```python
from build123d import *

# Parameters (mm, degrees)
BOSS_EXTRUDE1_DEPTH = 1828.8
THRU_HOLES_D        = 2.794


with BuildPart() as part:
    # Sketch1 → Boss-Extrude1 (new body)
    with BuildSketch(Plane(origin=(0, 0, 0), x_dir=(1, 0, 0), z_dir=(0, 1, 0))):
        with BuildLine():
            Line((-3.048, 13.208), (-3.048, 4.953))
            ThreePointArc((-3.048, 4.953), (-3.085197439, 4.863197439), (-3.175, 4.826))
            Line((-3.175, 4.826), (-4.826, 4.826))
            ThreePointArc((-4.826, 4.826), (-5.005605122, 4.751605122), (-5.08, 4.572))
            Line((-5.08, 4.572), (-5.08, 0))
            ThreePointArc((-5.08, 0), (-3.592102448, -3.592102448), (0, -5.08))
            Line((0, -5.08), (4.572, -5.08))
            ThreePointArc((4.572, -5.08), (4.751605122, -5.005605122), (4.826, -4.826))
            Line((4.826, -4.826), (4.826, -3.175))
            ThreePointArc((4.826, -3.175), (4.863197439, -3.085197439), (4.953, -3.048))
            Line((4.953, -3.048), (13.208, -3.048))
            ThreePointArc((13.208, -3.048), (13.746815367, -2.824815367), (13.97, -2.286))
            Line((13.97, -2.286), (13.97, 0.508))
            ThreePointArc((13.97, 0.508), (13.746815367, 1.046815367), (13.208, 1.27))
            Line((13.208, 1.27), (3.767428831, 1.27))
            ThreePointArc((3.767428831, 1.27), (3.625438515, 1.313394326), (3.531964529, 1.42875))
            ThreePointArc((3.531964529, 1.42875), (2.694076836, 2.694076836), (1.42875, 3.531964529))
            ThreePointArc((1.42875, 3.531964529), (1.313394326, 3.625438515), (1.27, 3.767428831))
            Line((1.27, 3.767428831), (1.27, 13.208))
            ThreePointArc((1.27, 13.208), (1.046815367, 13.746815367), (0.508, 13.97))
            Line((0.508, 13.97), (-2.286, 13.97))
            ThreePointArc((-2.286, 13.97), (-2.824815367, 13.746815367), (-3.048, 13.208))
        make_face()
    extrude(amount=BOSS_EXTRUDE1_DEPTH)

    # THRU HOLES (through all)
    with Locations(Plane(origin=(0, 1828.8, 0), x_dir=(1, 0, 0), z_dir=(0, 1, 0))):
        with Locations((0, 0)):
            Hole(THRU_HOLES_D / 2)


solid = part.part
```
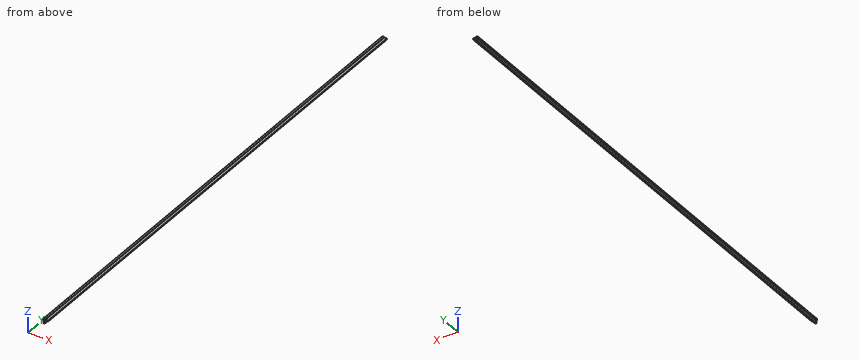
Input: part model. Units: mm. Frame: model coordinates. Give positions to 0.01 mm unless a question says otherwise; leave off trailing zeros. Order: outer loops, then holes, each group sorted by start corner. A loop starts at its lowest first (then second) coordinate and runs counter-clockwise, first axis right, second up. Notation, with made-up numbers: M 72,53.5 L 103,53.5 A17 ccw 103,72.5 Z; hole C -22,-27.5 d5. An arc over 180 degrees is marked long. Return JSON: item names as keys, results as strings.
1) Line query: L1, parallel to Z at x = 0, y = 1240.5; L2, parallel to X at y = 1159, z = -4.25; L3, parallel to Z at x = -3.75, y = 705.5. Output: solid intervals per line, ascending. Write a range as [from, to].
Taken from the geometry:
{"L1": "z = [-13.97, -1.4], [1.4, 5.08]", "L2": "x = [-5.08, 1.27]", "L3": "z = [-4.83, 3.43]"}
2) Section query A-A on y = 513.5. Output: boundary loops of the cut face in (x, z) (3 decimals).
Taken from the geometry:
{"outline": "M -5.08,-4.572 A0.254 ccw -4.826,-4.826 L -3.175,-4.826 A0.127 cw -3.048,-4.953 L -3.048,-13.208 A0.762 ccw -2.286,-13.97 L 0.508,-13.97 A0.762 ccw 1.27,-13.208 L 1.27,-3.767 A0.254 cw 1.429,-3.532 A3.81 ccw 3.532,-1.429 A0.254 cw 3.767,-1.27 L 13.208,-1.27 A0.762 ccw 13.97,-0.508 L 13.97,2.286 A0.762 ccw 13.208,3.048 L 4.953,3.048 A0.127 cw 4.826,3.175 L 4.826,4.826 A0.254 ccw 4.572,5.08 L 0,5.08 A5.08 ccw -5.08,0 Z; hole C 0,0 d2.794"}
3) Contact query for flat-ended pins moving along their axis: pin 1 (1.5 mm diameter, centred on x = 6.5, y = 928.5, fed in from -Z); pin 2 (4.5 mm diameter, centred on y = 1243, z = -8.5, fed in from +X); pin 3 (6.5 mm diameter, centred on x = 9.5, y = 752, fed in from +Z); pin 4 (8 mm diameter, centred on x = 6, z = -6.5, fed in from +Y). Output: stop coordinate, or through.
Taken from the geometry:
{"pin 1": "stops at z = -1.27", "pin 2": "stops at x = 1.27", "pin 3": "stops at z = 3.05", "pin 4": "passes through"}
4) Section query B-B on x = 8.25. Output: boundary loops of the cut face in (y, z).
Taken from the geometry:
{"outline": "M 0,-1.27 L 1828.8,-1.27 L 1828.8,3.05 L 0,3.05 Z"}
